Here's how the part is built. I have some questions about the finished solid (model axes, mm). Round coordinates to 2 decimals unless told otherwise and drop trailing zeros. Order: outer loops, then holes, each group sorted by start corner. A loop starts at its lowest first (then second) coordinate and runs counter-clockwise, first axis right, second up. Notation, with made-up numbers: (58, 75.5) -> (76, 75.5) arc R23 cw to (76, 83.5) -> close; hole circle Ø11 at (12, 31). An arc over 180 degrees is marked (long way). Use a Markdown table: item, result. Add a question column.
(1) I want a section at A-A, the plane z = -28. Please give me the cut outline in (x, y), then the cut area to 3 significant figures.
(2) If I drill on probe 1 along X at (y, z) = (1.45, 45); probe 2 along X at (y, z) = (0.9, 28); probe 3 along X at (y, z) = (2, -18.5), over which ranges is the centre line in solid material (lowest first)?
(3) I want a section at C-C, the plane z = 45. Please give me the cut outline in (x, y), then the cut area to 3 significant figures.
(4) I want a section at B-B, the plane x = -55. Please give me the cut outline in (y, z), then the cut area to 3 significant figures.
(5) I want a section at D-D, the plane z = 18.5. Please give me the cut outline in (x, y), then the cut area to 3 significant figures.
from build123d import *

# Parameters (mm, degrees)
SKETCH2_W           = 120
SKETCH2_H           = 100
BOSS_EXTRUDE1_DEPTH = 4
SKETCH3_R           = 1.5
CUT_EXTRUDE1_DEPTH  = 5
SKETCH4_R           = 1.65
CUT_EXTRUDE2_DEPTH  = 5
SKETCH6_R           = 1.6
CUT_EXTRUDE3_DEPTH  = 5
CUT_EXTRUDE4_DEPTH  = 21


with BuildPart() as part:
    # Sketch2 → Boss-Extrude1 (new body)
    with BuildSketch(Plane(origin=(0, 0, 0), x_dir=(1, 0, 0), z_dir=(0, 1, 0))):
        Rectangle(SKETCH2_W, SKETCH2_H)
    extrude(amount=BOSS_EXTRUDE1_DEPTH)

    # Sketch3 → Cut-Extrude1 (cut)
    with BuildSketch(Plane(origin=(0, 4, 0), x_dir=(1, 0, 0), z_dir=(0, 1, 0))):
        with Locations(Location((-55, 45, 0), (0, 0, 270))):
            Circle(SKETCH3_R)
        with Locations(Location((55, 45, 0), (0, 0, 270))):
            Circle(SKETCH3_R)
        with Locations(Location((55, -45, 0), (0, 0, 270))):
            Circle(SKETCH3_R)
        with Locations(Location((-55, -45, 0), (0, 0, 270))):
            Circle(SKETCH3_R)
    extrude(amount=-CUT_EXTRUDE1_DEPTH, mode=Mode.SUBTRACT)

    # Sketch4 → Cut-Extrude2 (cut)
    with BuildSketch(Plane(origin=(0, 4, 0), x_dir=(1, 0, 0), z_dir=(0, 1, 0))):
        with Locations(Location((-38, 37.5, 0), (0, 0, 270))):
            Circle(SKETCH4_R)
        with Locations(Location((-4, 37.5, 0), (0, 0, 270))):
            Circle(SKETCH4_R)
        with Locations(Location((38, 15.5, 0), (0, 0, 270))):
            Circle(SKETCH4_R)
        with Locations(Location((38, -18.5, 0), (0, 0, 270))):
            Circle(SKETCH4_R)
        with Locations(Location((-28.5, 28, 0), (0, 0, 270))):
            Circle(SKETCH4_R)
        with Locations(Location((-38, 18.5, 0), (0, 0, 270))):
            Circle(SKETCH4_R)
        with Locations(Location((-47.5, 28, 0), (0, 0, 270))):
            Circle(SKETCH4_R)
        with Locations(Location((5.5, 28, 0), (0, 0, 270))):
            Circle(SKETCH4_R)
        with Locations(Location((-4, 18.5, 0), (0, 0, 270))):
            Circle(SKETCH4_R)
        with Locations(Location((-13.5, 28, 0), (0, 0, 270))):
            Circle(SKETCH4_R)
        with Locations(Location((47.5, 6, 0), (0, 0, 270))):
            Circle(SKETCH4_R)
        with Locations(Location((38, -3.5, 0), (0, 0, 270))):
            Circle(SKETCH4_R)
        with Locations(Location((28.5, 6, 0), (0, 0, 270))):
            Circle(SKETCH4_R)
        with Locations(Location((47.5, -28, 0), (0, 0, 270))):
            Circle(SKETCH4_R)
        with Locations(Location((38, -37.5, 0), (0, 0, 270))):
            Circle(SKETCH4_R)
        with Locations(Location((28.5, -28, 0), (0, 0, 270))):
            Circle(SKETCH4_R)
    extrude(amount=-CUT_EXTRUDE2_DEPTH, mode=Mode.SUBTRACT)

    # Sketch6 → Cut-Extrude3 (cut)
    with BuildSketch(Plane(origin=(0, 4, 0), x_dir=(1, 0, 0), z_dir=(0, 1, 0))):
        with Locations(Location((5, 0, 0), (0, 0, 270))):
            Circle(SKETCH6_R)
        with Locations(Location((-5, 0, 0), (0, 0, 270))):
            Circle(SKETCH6_R)
    extrude(amount=-CUT_EXTRUDE3_DEPTH, mode=Mode.SUBTRACT)

    # Sketch7 → Cut-Extrude4 (cut)
    with BuildSketch(Plane(origin=(0, 4, 0), x_dir=(1, 0, 0), z_dir=(0, 1, 0))):
        with BuildLine():
            Line((-4, 39.15), (2, 39.15))
            ThreePointArc((2, 39.15), (3.65, 37.5), (2, 35.85))
            Line((2, 35.85), (-4, 35.85))
            ThreePointArc((-4, 35.85), (-5.65, 37.5), (-4, 39.15))
        make_face()
        with BuildLine():
            Line((5.5, 29.65), (11.5, 29.65))
            ThreePointArc((11.5, 29.65), (13.15, 28), (11.5, 26.35))
            Line((11.5, 26.35), (5.5, 26.35))
            ThreePointArc((5.5, 26.35), (3.85, 28), (5.5, 29.65))
        make_face()
        with BuildLine():
            Line((-4, 20.15), (2, 20.15))
            ThreePointArc((2, 20.15), (3.65, 18.5), (2, 16.85))
            Line((2, 16.85), (-4, 16.85))
            ThreePointArc((-4, 16.85), (-5.65, 18.5), (-4, 20.15))
        make_face()
        with BuildLine():
            Line((-13.5, 29.65), (-7.5, 29.65))
            ThreePointArc((-7.5, 29.65), (-5.85, 28), (-7.5, 26.35))
            Line((-7.5, 26.35), (-13.5, 26.35))
            ThreePointArc((-13.5, 26.35), (-15.15, 28), (-13.5, 29.65))
        make_face()
        with BuildLine():
            Line((36.35, 15.5), (36.35, 21.5))
            ThreePointArc((36.35, 21.5), (38, 23.15), (39.65, 21.5))
            Line((39.65, 21.5), (39.65, 15.5))
            ThreePointArc((39.65, 15.5), (38, 13.85), (36.35, 15.5))
        make_face()
        with BuildLine():
            Line((45.85, 6), (45.85, 12))
            ThreePointArc((45.85, 12), (47.5, 13.65), (49.15, 12))
            Line((49.15, 12), (49.15, 6))
            ThreePointArc((49.15, 6), (47.5, 4.35), (45.85, 6))
        make_face()
        with BuildLine():
            Line((36.35, -3.5), (36.35, 2.5))
            ThreePointArc((36.35, 2.5), (38, 4.15), (39.65, 2.5))
            Line((39.65, 2.5), (39.65, -3.5))
            ThreePointArc((39.65, -3.5), (38, -5.15), (36.35, -3.5))
        make_face()
        with BuildLine():
            Line((26.85, 6), (26.85, 12))
            ThreePointArc((26.85, 12), (28.5, 13.65), (30.15, 12))
            Line((30.15, 12), (30.15, 6))
            ThreePointArc((30.15, 6), (28.5, 4.35), (26.85, 6))
        make_face()
    extrude(amount=-CUT_EXTRUDE4_DEPTH, mode=Mode.SUBTRACT)


solid = part.part
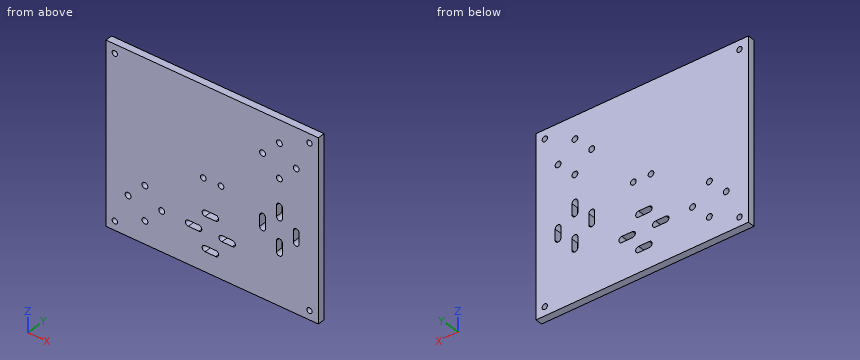
Taken from the geometry:
| question | item | result |
|---|---|---|
| 1 | outline | (-60, 0) -> (-49.15, 0) -> (-49.15, 4) -> (-60, 4) -> close; (-45.85, 0) -> (-30.15, 0) -> (-30.15, 4) -> (-45.85, 4) -> close; (-26.85, 0) -> (-15.15, 0) -> (-15.15, 4) -> (-26.85, 4) -> close; (-5.85, 0) -> (3.85, 0) -> (3.85, 4) -> (-5.85, 4) -> close; (13.15, 0) -> (60, 0) -> (60, 4) -> (13.15, 4) -> close |
| 1 | area | 379 mm2 |
| 2 | probe 1 | x = -60 to -56.5, -53.5 to 53.5, 56.5 to 60 |
| 2 | probe 2 | x = -60 to 26.85, 30.15 to 45.85, 49.15 to 60 |
| 2 | probe 3 | x = -60 to -39.65, -36.35 to -5.65, 3.65 to 36.35, 39.65 to 60 |
| 3 | outline | (-60, 0) -> (-56.5, 0) -> (-56.5, 4) -> (-60, 4) -> close; (-53.5, 0) -> (53.5, 0) -> (53.5, 4) -> (-53.5, 4) -> close; (56.5, 0) -> (60, 0) -> (60, 4) -> (56.5, 4) -> close |
| 3 | area | 456 mm2 |
| 4 | outline | (0, -50) -> (4, -50) -> (4, -46.5) -> (0, -46.5) -> close; (0, -43.5) -> (4, -43.5) -> (4, 43.5) -> (0, 43.5) -> close; (0, 46.5) -> (4, 46.5) -> (4, 50) -> (0, 50) -> close |
| 4 | area | 376 mm2 |
| 5 | outline | (-60, 0) -> (36.35, 0) -> (36.35, 4) -> (-60, 4) -> close; (39.65, 0) -> (60, 0) -> (60, 4) -> (39.65, 4) -> close |
| 5 | area | 467 mm2 |
